Answer from the drawing. Dimensions are ordinates in mm from the lowest x, y and z of the part. Give positions to 0.01 mm unless a question says otherwise; leave off trailing zeros. Loops run counter-clockwise (first coordinate to the right, second up) from the corner with the lowest first, then second, coordinate; pieces in that order, holes last.
(1) Straight lines are drawn through the part: probe 1 along X at (y, z) = (0.8, 41); probe 2 along X at (y, z) = (1.7, 20.5); probe 3 along X at (y, z) = (1, 34). For each, find the intervals that lie inside material, in ascending order.
(2) Find section A-A, the plane z = 41. Write down the section's boundary in (x, y).
(3) Find section C-C, the plane y = 1.8. State how many separate pieces and enclosed holes the cut face has, then the cut area to 3 significant figures.
(4) This flat-tipped pin is pushed along its axis until it touches: P1, Ø2, axis at x = 5, z = 10, coming from the -Y side. Where does it stop, or does it pass through?
(5) Find section B-B, the plane x = 69. Write down the section's boundary in (y, z).
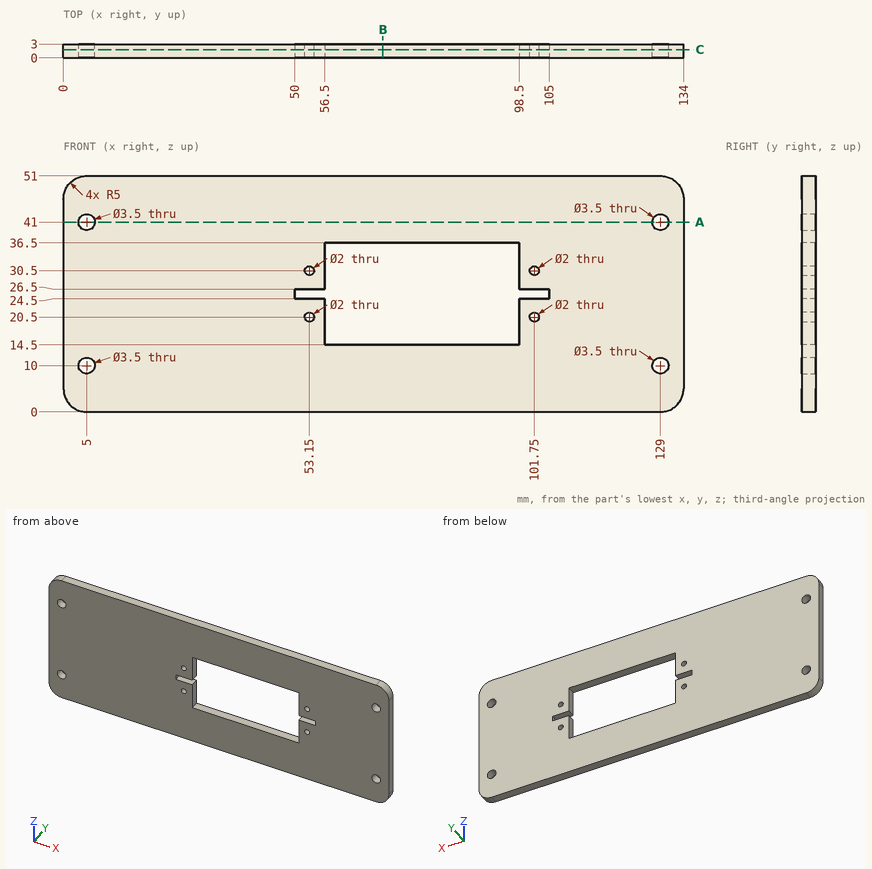
Entries:
1. probe 1: x = 0 to 3.25, 6.75 to 127.25, 130.75 to 134
1. probe 2: x = 0 to 52.15, 54.15 to 56.5, 98.5 to 100.75, 102.75 to 134
1. probe 3: x = 0 to 56.5, 98.5 to 134
2. outline: (0, 0) - (3.25, 0) - (3.25, 3) - (0, 3) - close; (6.75, 0) - (127.25, 0) - (127.25, 3) - (6.75, 3) - close; (130.75, 0) - (134, 0) - (134, 3) - (130.75, 3) - close
3. separate pieces: 1
3. enclosed holes: 9
3. area: 5,810 mm2
4. P1: passes through
5. outline: (0, 0) - (3, 0) - (3, 14.5) - (0, 14.5) - close; (0, 36.5) - (3, 36.5) - (3, 51) - (0, 51) - close
